Check sheet for the modelled part. Datum: model origin and axes. Units: mm. A direction names the side the tool comes from. Round coordinates to 2 decimals unless told otherwise and drop trailing zeros. Write each loop counter-clockwise with the first axis right and the second up, starting at its lowest first coordinate (ties: lowest second). Pieces come first, ordered by that corner, then holes. Notation, with made-up numbers: (1, 56) -> (30, 56) arc R15 cw to (30, 62) -> close; hole circle Ø10 at (-35, -14). An arc over 180 degrees is marked (long way). One line per item, written item: value.
from build123d import *

# Parameters (mm, degrees)
SKETCH_1_W                = 150
SKETCH_1_H                = 160
EXTRUDE_1_DEPTH           = 5
SKETCH_2_R                = 1.75
CUT_EXTRUDE_1_DEPTH       = 110.772492001
SKETCH_3_R                = 1.75
CUT_EXTRUDE_2_DEPTH       = 110.772492001
SKETCH_4_R                = 2.55
CUT_EXTRUDE_3_DEPTH       = 7
FILLET_1_R                = 8
SKETCH_5_R                = 2.55
CUT_EXTRUDE_4_DEPTH       = 110.772492001
EXTRUDE_2_DEPTH           = 40
SKETCH_7_R                = 5
SKETCH_7_R_2              = 4.71820485
CUT_EXTRUDE_5_DEPTH       = 2
CUT_EXTRUDE_6_DEPTH       = 159.533908045
CUT_EXTRUDE_6_DEPTH_BACK  = 159.533908045
SKETCH_9_R                = 1.25
CUT_EXTRUDE_7_DEPTH       = 159.533908045
CUT_EXTRUDE_7_DEPTH_BACK  = 159.533908045
SKETCH_11_R               = 3
CUT_EXTRUDE_8_DEPTH       = 130.031004026
SKETCH_12_R               = 1.25
EXTRUDE_3_DEPTH           = 6
SKETCH_13_W               = 52
SKETCH_13_H               = 52
CUT_EXTRUDE_9_DEPTH       = 2
CUT_EXTRUDE_10_DEPTH      = 130.031004026
CUT_EXTRUDE_10_DEPTH_BACK = 5
SKETCH_14_R               = 1.2
FILLET_2_R                = 2
FILLET_3_R                = 5
CHAMFER_1_SIZE            = 0.2


with BuildPart() as part:
    # 草图1 → 凸台-拉伸1 (new body)
    with BuildSketch(Plane.XY):
        Rectangle(SKETCH_1_W, SKETCH_1_H)
    extrude(amount=EXTRUDE_1_DEPTH)

    # 草图2 → 切除-拉伸1 (cut, through all)
    with BuildSketch(Plane.XY.offset(5)):
        with Locations((-20, -15)):
            Circle(SKETCH_2_R)
        with Locations((20, -15)):
            Circle(SKETCH_2_R)
        with Locations((20, -55)):
            Circle(SKETCH_2_R)
        with Locations((-20, -55)):
            Circle(SKETCH_2_R)
    extrude(amount=-CUT_EXTRUDE_1_DEPTH, mode=Mode.SUBTRACT)

    # 草图3 → 切除-拉伸2 (cut, through all)
    with BuildSketch(Plane.XY.offset(5)):
        with Locations((46, 20)):
            Circle(SKETCH_3_R)
        with Locations((46, -50)):
            Circle(SKETCH_3_R)
        with Locations((-46, -50)):
            Circle(SKETCH_3_R)
        with Locations((-46, 20)):
            Circle(SKETCH_3_R)
    extrude(amount=-CUT_EXTRUDE_2_DEPTH, mode=Mode.SUBTRACT)

    # 草图4 → 切除-拉伸3 (cut)
    with BuildSketch(Plane.XY.offset(5)):
        with Locations((-67, -72)):
            Circle(SKETCH_4_R)
        with Locations((67, -72)):
            Circle(SKETCH_4_R)
        with Locations((-67, 62)):
            Circle(SKETCH_4_R)
        with Locations((67, 62)):
            Circle(SKETCH_4_R)
    extrude(amount=-CUT_EXTRUDE_3_DEPTH, mode=Mode.SUBTRACT)

    # 圆角1
    fillet_1_edges = [part.edges().sort_by_distance(p)[0] for p in [
        (75, -80, 2.5),
        (-75, -80, 2.5),
        (-75, 80, 2.5),
        (75, 80, 2.5),
    ]]
    fillet(fillet_1_edges, radius=FILLET_1_R)

    # 草图5 → 切除-拉伸4 (cut, through all)
    with BuildSketch(Plane.XY.offset(5)):
        with Locations((0, 65)):
            Circle(SKETCH_5_R)
    extrude(amount=-CUT_EXTRUDE_4_DEPTH, mode=Mode.SUBTRACT)

    # 草图6 → 凸台-拉伸2 (add, symmetric)
    with BuildSketch(Plane(origin=(0, 0, 0), x_dir=(0, 0, -1), z_dir=(1, 0, 0))):
        Polygon((-5, 80), (-5, 38), (-68, 38), (-68, 42), (-8, 42), (-8, 80), align=None)
    extrude(amount=EXTRUDE_2_DEPTH, both=True)

    # 草图7 → 切除-拉伸5 (cut)
    with BuildSketch(Plane.XY.offset(5)):
        with Locations((67, 62)):
            Circle(SKETCH_7_R)
        with Locations((-67, 62)):
            Circle(SKETCH_7_R)
        with Locations((67, -72)):
            Circle(SKETCH_7_R_2)
        with Locations((-67, -72)):
            Circle(SKETCH_7_R)
    extrude(amount=-CUT_EXTRUDE_5_DEPTH, mode=Mode.SUBTRACT)

    # 草图9 → 切除-拉伸6 (cut, two sides: drawn at the far end of the back side and taken through both)
    with BuildSketch(Plane(origin=(0, 42, 0), x_dir=(1, 0, 0), z_dir=(0, 1, 0)).offset(-CUT_EXTRUDE_6_DEPTH_BACK)):
        with Locations(Location((22.5, -55, 0), (0, 0, 270))):
            Circle(SKETCH_9_R)
        with Locations(Location((-22.5, -55, 0), (0, 0, 270))):
            Circle(SKETCH_9_R)
    extrude(amount=CUT_EXTRUDE_6_DEPTH + CUT_EXTRUDE_6_DEPTH_BACK, mode=Mode.SUBTRACT)

    # 草图10 → 切除-拉伸7 (cut, two sides: drawn at the far end of the back side and taken through both)
    with BuildSketch(Plane(origin=(0, 42, 0), x_dir=(1, 0, 0), z_dir=(0, 1, 0)).offset(-CUT_EXTRUDE_7_DEPTH_BACK)):
        with BuildLine():
            Line((10, -30), (-10, -30))
            ThreePointArc((-10, -30), (-20, -20), (-10, -10))
            Line((-10, -10), (10, -10))
            ThreePointArc((10, -10), (20, -20), (10, -30))
        make_face()
    extrude(amount=CUT_EXTRUDE_7_DEPTH + CUT_EXTRUDE_7_DEPTH_BACK, mode=Mode.SUBTRACT)

    # 草图11 → 切除-拉伸8 (cut, through all)
    with BuildSketch(Plane(origin=(0, 0, 0), x_dir=(-1, 0, 0), z_dir=(0, 0, -1))):
        with Locations((0, 65)):
            Circle(SKETCH_11_R)
    extrude(amount=-CUT_EXTRUDE_8_DEPTH, mode=Mode.SUBTRACT)

    # 草图12 → 凸台-拉伸3 (add)
    with BuildSketch(Plane.XY.offset(8)):
        with Locations(Location((18, 65, 0), (0, 0, 90))):
            Circle(SKETCH_12_R)
        with Locations(Location((-18, 65, 0), (0, 0, 180))):
            Circle(SKETCH_12_R)
    extrude(amount=EXTRUDE_3_DEPTH)

    # 草图13 → 切除-拉伸9 (cut)
    with BuildSketch(Plane.XY.offset(5)):
        with Locations((0, -35)):
            Rectangle(SKETCH_13_W, SKETCH_13_H)
    extrude(amount=-CUT_EXTRUDE_9_DEPTH, mode=Mode.SUBTRACT)

    # 草图14 → 切除-拉伸10 (cut, two sides: drawn at the far end of the back side and taken through both)
    with BuildSketch(Plane(origin=(0, 0, 0), x_dir=(-1, 0, 0), z_dir=(0, 0, -1)).offset(-CUT_EXTRUDE_10_DEPTH_BACK)):
        with Locations(Location((17, -5, 0), (0, 0, 180))):
            Circle(SKETCH_14_R)
        with Locations(Location((17, 56, 0), (0, 0, 180))):
            Circle(SKETCH_14_R)
        with Locations(Location((-17, 56, 0), (0, 0, 180))):
            Circle(SKETCH_14_R)
        with Locations(Location((-17, -5, 0), (0, 0, 180))):
            Circle(SKETCH_14_R)
    extrude(amount=CUT_EXTRUDE_10_DEPTH + CUT_EXTRUDE_10_DEPTH_BACK, mode=Mode.SUBTRACT)

    # 圆角2
    fillet_2_edges = [part.edges().sort_by_distance(p)[0] for p in [
        (26, -9, 4),
        (26, -61, 4),
        (-26, -61, 4),
        (-26, -9, 4),
    ]]
    fillet(fillet_2_edges, radius=FILLET_2_R)

    # 圆角3
    fillet_3_edges = [part.edges().sort_by_distance(p)[0] for p in [
        (-40, 40, 68),
        (40, 40, 68),
    ]]
    fillet(fillet_3_edges, radius=FILLET_3_R)

    # 倒角1
    chamfer_1_edges = [part.edges().sort_by_distance(p)[0] for p in [
        (18, 63.75, 14),
        (-16.75, 65, 14),
    ]]
    chamfer(chamfer_1_edges, length=CHAMFER_1_SIZE)


solid = part.part
Item 1: Release check for a two-part mould opening along Y. For faces 1 (the cylindrical face through (-72.719, -77.594, 2.535)), 2 (the cylindrical face through (20, 40, 20)), 3 (the flat face through (0, -35, 3)) record: pulls with the +Y half, pulls with the -Y half, needs draft (parallel to the pull), parting line crosses it, or undercut.
Result set:
face 1: pulls with the -Y half
face 2: needs draft
face 3: undercut
Item 2: Depth check by flat-ended pin: pin 1 (2 mm diameter, centred on x = 20, y = -15, fed in from -Z); pin 2 (3 mm diameter, centred on x = -69, y = -72, fed in from +Z); pin 3 (2.5 mm diameter, centred on x = 18.5, y = 65, fed in from +Z); pin 4 (1 mm diameter, centred on x = 27.5, z = 9.5, fed in from +Y). Enter the tip coordinate at first touch or a pass-through.
Result set:
pin 1: through
pin 2: z = 3
pin 3: z = 14
pin 4: y = 42
Item 3: Tool access check on faces 4 (the flat face through (-40, 40, 25)), 5 (the flat face through (40, 40, 25)), 6 (the flat face through (-1, -80, 2)), 7 (the flat face through (-65, -74, 3)). Record the directions out of +Z, -Z, +X, -X, +Y, -Y that give a thin tool (end or side, any length) a straight path to the whole face; none if there is none.
Result set:
face 4: +Z, -X, +Y, -Y
face 5: +Z, +X, +Y, -Y
face 6: +Z, -Z, +X, -X, -Y
face 7: +Z
Item 4: Material ranges on line 1 along Y through (x, z) = (17, 1.05); line 2 along Z through (x, y) = (-22.5, 41.15); line 3 along Z through (x, y) = (32, -34), recorded low to high.
Result set:
line 1: -80 to -6.2, -3.8 to 54.8, 57.2 to 80
line 2: 0 to 53.75, 56.25 to 68
line 3: 0 to 5
Item 5: Sectioned sample at A-A (x = -6.5). Enter the section's corners in (y, z), then the cut area to 3 significant figures.
Result set:
outline: (-80, 0) -> (80, 0) -> (80, 8) -> (42, 8) -> (42, 10) -> (38, 10) -> (38, 5) -> (-9, 5) -> (-9, 3) -> (-61, 3) -> (-61, 5) -> (-80, 5) -> close; (38, 30) -> (42, 30) -> (42, 68) -> (38, 68) -> close
area: 982 mm^2
Item 6: Sectioned sample at D-D (x = 50.5). Enter the section's corners in (y, z).
Result set:
outline: (-80, 0) -> (80, 0) -> (80, 5) -> (-80, 5) -> close
Item 7: Sectioned sample at B-B (z = 20). Enter the section's corners in (x, y).
Result set:
outline: (-40, 38) -> (-20, 38) -> (-20, 42) -> (-40, 42) -> close; (20, 38) -> (40, 38) -> (40, 42) -> (20, 42) -> close
Item 8: Sectioned sample at C-C (y = 48). Enter the section's corners in (x, z).
Result set:
outline: (-75, 0) -> (75, 0) -> (75, 5) -> (40, 5) -> (40, 8) -> (-40, 8) -> (-40, 5) -> (-75, 5) -> close
